Part model, mm, in its own coordinate system. Coordinates: 2 decimals unless noted, no trailing zeros. Loops run counter-clockwise (first coordinate to the right, second up) from the corner with the lowest first, then second, coordinate; pieces in that order, holes last. Notation, with made-up numbers: (72.5, -0.5) - (122.5, -0.5) arc R17 cw to (122.5, 19.5) - close; hole circle Ø7 at (89, 66.25). An arc over 180 degrees is marked (long way). Use a Markdown table: item, result. Add a question column.
1. Band-saw the part on D-D, the plane x = 306. Give the cut face in (y, z), plus the area to 3 significant figures.
2. Pull direction X, two halves, no side cores. Call faces 1 (the flat face through (318.268, 97.266, 0.986)), 2 (the cylindrical face through (304.7, 30.607, 0.986)), 3 (the cylindrical face through (27.67, 15.85, 1.01)): pulls with the +X half, pulls with the -X half, needs draft (parallel to the pull), parting line crosses it, or undercut.
3. Wall check: probe 1 along X at (y, z) = (145, 0.65); probe 2 along X at (y, z) = (9.5, 0.35); probe 3 along Y at (x, z) = (121.5, 0.9). Give the ranges that are in metal, low to high. Write a range as [from, to].
4. Band-saw the part on B-B, the plane z = 1.65. Give the cut face in (x, y), plus the area to 3 significant figures.
5. Band-saw the part on C-C, the plane y = 145. Give the cut face in (x, z).
6. Band-saw the part on A-A, the plane x = 110. Give the cut face in (y, z).
from build123d import *

# Parameters (mm, degrees)
SKETCH1_R           = 3.5
SKETCH1_R_2         = 4.5
BOSS_EXTRUDE1_DEPTH = 2
FILLET1_R           = 30
FILLET2_R           = 10


with BuildPart() as part:
    # Sketch1 → Boss-Extrude1 (new body)
    with BuildSketch(Plane.XY):
        Polygon((0, 0), (98.729357602, 158), (293.729357602, 158), (357.565501284, 0), align=None)
        with Locations((284.960746883, 145)):
            Circle(SKETCH1_R, mode=Mode.SUBTRACT)
        with Locations((305.675867386, 35)):
            Circle(SKETCH1_R_2, mode=Mode.SUBTRACT)
        with Locations((63.141671434, 35)):
            Circle(SKETCH1_R_2, mode=Mode.SUBTRACT)
        with Locations((123.141671434, 13)):
            Circle(SKETCH1_R_2, mode=Mode.SUBTRACT)
        with Locations((223.141671434, 13)):
            Circle(SKETCH1_R_2, mode=Mode.SUBTRACT)
        with BuildLine():
            Line((105.935375271, 148.5), (123.935375271, 148.5))
            ThreePointArc((123.935375271, 148.5), (127.435375271, 145), (123.935375271, 141.5))
            Line((123.935375271, 141.5), (105.935375271, 141.5))
            ThreePointArc((105.935375271, 141.5), (102.435375271, 145), (105.935375271, 148.5))
        make_face(mode=Mode.SUBTRACT)
    extrude(amount=BOSS_EXTRUDE1_DEPTH)

    # Fillet1
    fillet1_edges = [part.edges().sort_by_distance(p)[0] for p in [
        (0, 0, 1),
        (357.565501284, 0, 1),
    ]]
    fillet(fillet1_edges, radius=FILLET1_R)

    # Fillet2
    fillet2_edges = [part.edges().sort_by_distance(p)[0] for p in [
        (98.729357602, 158, 1),
        (293.729357602, 158, 1),
    ]]
    fillet(fillet2_edges, radius=FILLET2_R)


solid = part.part
Geometry check:
| question | item | result |
|---|---|---|
| 1 | outline | (0, 0) - (30.51, 0) - (30.51, 2) - (0, 2) - close; (39.49, 0) - (127.63, 0) - (127.63, 2) - (39.49, 2) - close |
| 1 | area | 237 mm^2 |
| 2 | face 1 | pulls with the +X half |
| 2 | face 2 | undercut |
| 2 | face 3 | pulls with the -X half |
| 3 | probe 1 | x = [90.61, 102.44], [127.44, 281.46], [288.46, 298.98] |
| 3 | probe 2 | x = [32.22, 120.31], [125.97, 220.31], [225.97, 334.99] |
| 3 | probe 3 | y = [0, 8.81], [17.19, 141.5], [148.5, 158] |
| 4 | outline | (28.68, 45.9) arc R30 ccw to (54.12, 0) - (313.09, 0) arc R30 ccw to (340.9, 41.24) - (296.26, 151.75) arc R10 ccw to (286.98, 158) - (104.27, 158) arc R10 ccw to (95.79, 153.3) - close; hole circle Ø9 at (63.14, 35); hole (105.94, 141.5) - (123.94, 141.5) arc R3.5 ccw to (123.94, 148.5) - (105.94, 148.5) arc R3.5 ccw to start; hole circle Ø9 at (123.14, 13); hole circle Ø9 at (223.14, 13); hole circle Ø7 at (284.96, 145); hole circle Ø9 at (305.68, 35) |
| 4 | area | 42,100 mm^2 |
| 5 | outline | (90.61, 0) - (102.44, 0) - (102.44, 2) - (90.61, 2) - close; (127.44, 0) - (281.46, 0) - (281.46, 2) - (127.44, 2) - close; (288.46, 0) - (298.98, 0) - (298.98, 2) - (288.46, 2) - close |
| 6 | outline | (0, 0) - (141.5, 0) - (141.5, 2) - (0, 2) - close; (148.5, 0) - (158, 0) - (158, 2) - (148.5, 2) - close |
